Verification items for the finished model (mm, model axes). Face numbers are marked on the shaded views. A direction names the side the tool comes from. Round coordinates to 2 decimals unless told otherwise and drop trailing zeros. Write each loop counter-clockwise with the first axis right and the second up, starting at its lowest first coordinate (ties: lowest second). Pieces come first, ordered by that corner, then holes.
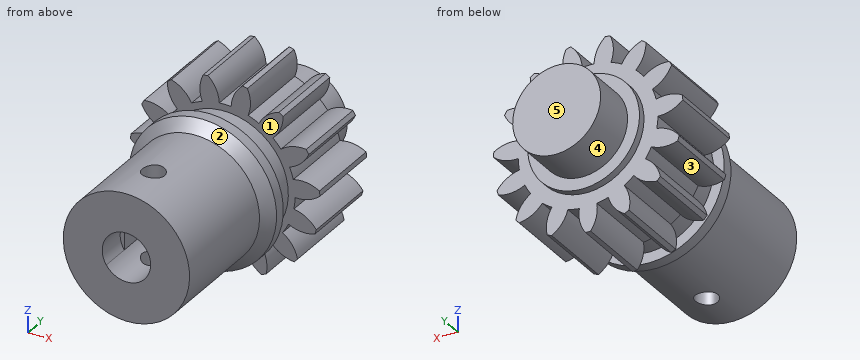
from build123d import *
from build123d.topology import SkipClean

# Parameters (mm, degrees)
RESSALTO_EXTRUS_O1_START   = -10.4
RESSALTO_EXTRUS_O1_DEPTH   = 10.4
PADR_OCIRCULAR1_COUNT      = 15
CORTE_EXTRUS_O1_DEPTH      = 22
ESBO_O4_R                  = 3.25
CORTE_EXTRUS_O2_DEPTH      = 4
CORTE_EXTRUS_O4_DEPTH      = 44.317435995
CORTE_EXTRUS_O4_DEPTH_BACK = 44.317435995
ESBO_O7_R                  = 1.5


with BuildPart() as part:
    # Esboço1 → Revolução1 (revolve)
    with BuildSketch(Plane.XY, mode=Mode.PRIVATE) as revolu_o1_sk:
        Polygon((0, 0), (0, 39.4), (5.9, 39.4), (5.9, 33.4), (7.5, 33.4), (7.5, 32.4), (9.374, 32.4), (9.374, 22), (8.47, 22), (8.47, 18.51), (9.9, 18.51), (9.9, 17.01), (8.47, 15.58), (8.47, 0), align=None)
    revolve(revolu_o1_sk.sketch.rotate(Axis((0, 0, 0), (0, 1, 0)), 90), axis=Axis((0, 0, 0), (0, 1, 0)))

    # Esboço2 → Ressalto-extrusão1 (add)
    with BuildSketch(Plane(origin=(0, 32.4, 0), x_dir=(1, 0, 0), z_dir=(0, 1, 0)).offset(RESSALTO_EXTRUS_O1_START)):
        with BuildLine():
            Line((-0.337, 12.746), (0.337, 12.746))
            ThreePointArc((0.337, 12.746), (1.105703178, 11.108702403), (1.167644885, 9.300993572))
            ThreePointArc((1.167644885, 9.300993572), (0, 9.374), (-1.167644885, 9.300993572))
            ThreePointArc((-1.167644885, 9.300993572), (-1.105703178, 11.108702403), (-0.337, 12.746))
        make_face()
    ressalto_extrus_o1 = extrude(amount=RESSALTO_EXTRUS_O1_DEPTH)

    # PadrãoCircular1: Ressalto-extrusão1 ×15 about axis
    padr_ocircular1_axis = Axis((0, 0, 0), (0, 1, 0))
    for i in range(1, PADR_OCIRCULAR1_COUNT):
        add(ressalto_extrus_o1.rotate(padr_ocircular1_axis, i * 360 / PADR_OCIRCULAR1_COUNT))

    # Esboço3 → Corte-extrusão1 (cut)
    with BuildSketch(Plane.XZ):
        with BuildLine():
            Line((2.65, 1.881488772), (2.65, -1.881488772))
            ThreePointArc((2.65, -1.881488772), (-0.044028005, -3.249701761), (-2.7, -1.809005252))
            Line((-2.7, -1.809005252), (-2.7, 1.809005252))
            ThreePointArc((-2.7, 1.809005252), (-0.044028005, 3.249701761), (2.65, 1.881488772))
        make_face()
    extrude(amount=-CORTE_EXTRUS_O1_DEPTH, mode=Mode.SUBTRACT)

    # Esboço4 → Corte-extrusão2 (cut)
    with SkipClean():  # the faces are left unmerged after this step: merging them gives an invalid solid
        with BuildSketch(Plane.XZ):
            with Locations(Location((0, 0, 0), (0, 0, 270))):
                Circle(ESBO_O4_R)
        extrude(amount=-CORTE_EXTRUS_O2_DEPTH, mode=Mode.SUBTRACT)

    # Esboço7 → Corte-extrusão4 (cut, two sides: drawn at the far end of the back side and taken through both)
    with BuildSketch(Plane.XY.offset(-CORTE_EXTRUS_O4_DEPTH_BACK)):
        with Locations((0, 6)):
            Circle(ESBO_O7_R)
    extrude(amount=CORTE_EXTRUS_O4_DEPTH + CORTE_EXTRUS_O4_DEPTH_BACK, mode=Mode.SUBTRACT)


solid = part.part
Q1. Release check for a two-part mould opening along Y. For the marked faces 1, 2 and 3 record: released by +Y, released by -Y, zero draft, split by the parting line, or undercut.
Recorded:
face 1: undercut
face 2: released by -Y
face 3: zero draft
Q2. Material ranges on line 1 along X through (y, z) = (23.5, 9.5); line 2 along Y through (x, z) = (0, 4.9); line 3 along Y through (x, z) = (-4.5, 4.5), recorded low to high.
Recorded:
line 1: x = -7.73 to -5.48, -3.28 to -0.8, 0.8 to 3.28, 5.48 to 7.73
line 2: y = 0 to 4.5, 7.5 to 39.4
line 3: y = 0 to 33.4
Q3. Depth check by flat-ended pin: P1, Ø1.8, axis at y = 10, z = -0.5, coming from the +X side; P2, Ø1.6, axis at x = -0.5, z = 0.5, coming from the -Y side; P3, Ø6, axis at x = -1, z = 2, coming from the -Y side; P4, Ø2, axis at y = 24.5, z = -2, coming from the +X side. Enter the tip coordinate at first touch or a pass-through.
Recorded:
P1: stops at x = 8.47
P2: stops at y = 22
P3: stops at y = 0
P4: stops at x = 11.7
Q4. Sectioned sample at A-A (y = 6). Enter the section's corners in (x, z).
Recorded:
outline: (-2.7, -1.81) - (-2.7, 1.81) arc R3.25 cw to (-1.5, 2.88) - (-1.5, 8.34) arc R8.47 ccw to (-1.5, -8.34) - (-1.5, -2.88) arc R3.25 cw to start; (1.5, -8.34) arc R8.47 ccw to (1.5, 8.34) - (1.5, 2.88) arc R3.25 cw to (2.65, 1.88) - (2.65, -1.88) arc R3.25 cw to (1.5, -2.88) - close
Q5. Tool access check on the marked faces 4 and 5. Record the directions out of +Z, -Z, +X, -X, +Y, -Y that give a thin tool (end or side, any length) a straight path to the whole face; none if there is none.
Recorded:
face 4: +Y
face 5: +Z, -Z, +X, -X, +Y
